The drawing under review shows one solid part. Ordinate dimensions are in mm from its lowest x, y, z. Give positions to 0.01 mm unless a question says otherwise; leave off trailing zeros. Write each loop counter-clockwise with the first axis right and the second up, starting at its lowest first coordinate (ties: lowest second). Pieces come first, ordered by that corner, then holes. Notation, with made-up numbers: (8, -14) -> (50, -14) arc R11 cw to (50, 2) -> close; hole circle Ø1 at (17, -20). An arc over 180 degrees is marked (long way). Answer as a JSON object with one key per item and string values.
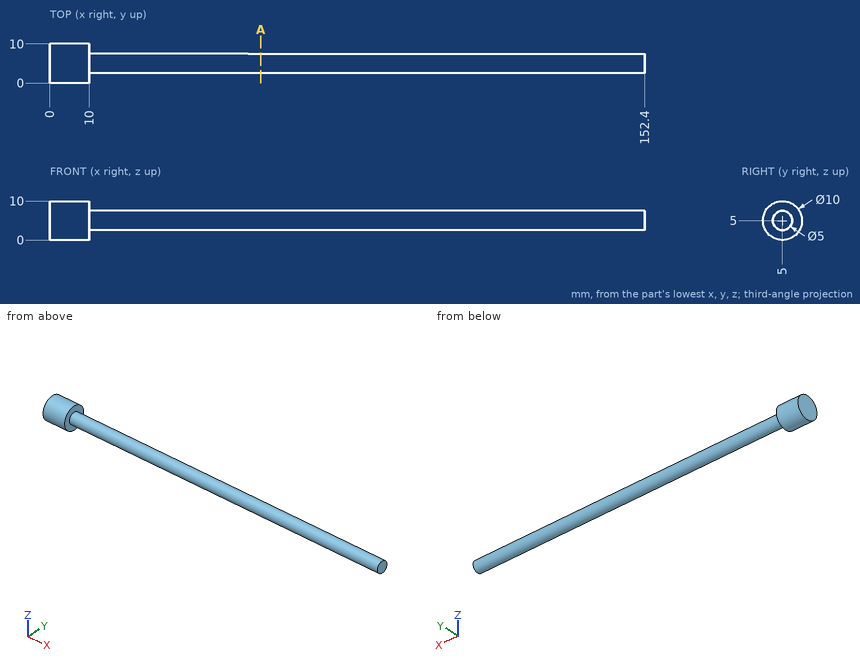
(1) Clearance check with flat-ended pins moving along their axes: pin 1 (4 mm diameter, centred on x = 131.5, z = 3, fed in from -Y); pin 2 (1.5 mm diameter, centred on y = 2.5, z = 3, fed in from -X); pin 3 (1 mm diameter, centred on y = 1, z = 3, fed in from +X); pin 4 (6 mm diameter, centred on x = 44, z = 2, fed in from +Y). State where each tip first meets the part, or that it passes through.
Here are the results:
{"pin 1": "stops at y = 2.5", "pin 2": "stops at x = 0", "pin 3": "stops at x = 10", "pin 4": "stops at y = 7.5"}
(2) For line 1 along X through (y, z) = (2.25, 1.5); line 2 along Y through (x, z) = (93, 4.75); line 3 along Z through (x, y) = (121, 6.5), list the stretches that pass through material, from the lowest coordinate up.
Here are the results:
{"line 1": "x = 0 to 10", "line 2": "y = 2.51 to 7.49", "line 3": "z = 3 to 7"}
(3) We need section A-A, the plane x = 54. State the section outline as (y, z) points.
Here are the results:
{"outline": "circle Ø5 at (5, 5)"}
